from build123d import *

# Parameters (mm, degrees)
BOSS_EXTRUDE1_DEPTH = 7
SKETCH4_R           = 11
CUT_EXTRUDE1_DEPTH  = 8
SKETCH7_R           = 4
CUT_EXTRUDE2_DEPTH  = 8


with BuildPart() as part:
    # Sketch2 → Boss-Extrude1 (new body)
    with BuildSketch(Plane.XY):
        with BuildLine():
            Line((0, 0), (45, 0))
            ThreePointArc((45, 0), (65, 20), (45, 40))
            Line((45, 40), (0, 40))
            ThreePointArc((0, 40), (-20, 20), (0, 0))
        make_face()
    extrude(amount=BOSS_EXTRUDE1_DEPTH)

    # Sketch4 → Cut-Extrude1 (cut, through all)
    with BuildSketch(Plane(origin=(0, 0, 0), x_dir=(-1, 0, 0), z_dir=(0, 0, -1))):
        with Locations((0, 20)):
            Circle(SKETCH4_R)
    extrude(amount=-CUT_EXTRUDE1_DEPTH, mode=Mode.SUBTRACT)

    # Sketch7 → Cut-Extrude2 (cut, through all)
    with BuildSketch(Plane.XY.offset(7)):
        with Locations((45, 20)):
            Circle(SKETCH7_R)
    extrude(amount=-CUT_EXTRUDE2_DEPTH, mode=Mode.SUBTRACT)


solid = part.part
Could you check a few things on this model? Use its own coordinates, in mm. Coordinates: 2 decimals unless noted, no trailing zeros. Order: outer loops, then holes, each group sorted by start corner. A loop starts at its lowest first (then second) coordinate and runs counter-clockwise, first axis right, second up.
Q1. Please list where these lines run through material, in increasing order: L1, parallel to Y at x = 45, z = 4; L2, parallel to Y at x = 0, z = 2; L3, parallel to X at y = 23.5, z = 5.
Q2. Will this pin go through, and if not, where does the flat tip stop? pin 1 (13 mm diameter, centred on x = 0, y = 20, fed in from -Z).
Q3. Thinking about a two-plate mould opening in Y: for faces 1 (the flat face through (23, 40, 3)), 2 (the flat face through (22, 0, 3)), 3 (the cylindrical face through (42.05, 22.7, 3.55)), which applies, released by +Y, released by -Y, zero draft, split by the parting line, or undercut?
Q4. Suppose I cut it at B-B on z = 1.75. Please give me the cut outline in (x, y), and give its area (3 significant figures).
Q5. Suppose I cut it at D-D on x = -7. Please give me the cut outline in (y, z) (3 decimals).
Q6. Suppose I cut it at C-C on y = 11.5. Please give me the cut outline in (x, z), and give its area (3 significant figures).
Q7. Suppose I cut it at A-A on y = 20. Please give me the cut outline in (x, z), and give its area (3 significant figures).
Answer:
1. L1: y = 0 to 16, 24 to 40
1. L2: y = 0 to 9, 31 to 40
1. L3: x = -19.69 to -10.43, 10.43 to 43.06, 46.94 to 64.69
2. pin 1: passes through
3. face 1: released by +Y
3. face 2: released by -Y
3. face 3: undercut
4. outline: (0, 0) - (45, 0) arc R20 ccw to (45, 40) - (0, 40) arc R20 ccw to start; hole circle Ø22 at (0, 20); hole circle Ø8 at (45, 20)
4. area: 2,630 mm2
5. outline: (1.265, 0) - (11.515, 0) - (11.515, 7) - (1.265, 7) - close; (28.485, 0) - (38.735, 0) - (38.735, 7) - (28.485, 7) - close
6. outline: (-18.1, 0) - (-6.98, 0) - (-6.98, 7) - (-18.1, 7) - close; (6.98, 0) - (63.1, 0) - (63.1, 7) - (6.98, 7) - close
6. area: 471 mm2
7. outline: (-20, 0) - (-11, 0) - (-11, 7) - (-20, 7) - close; (11, 0) - (41, 0) - (41, 7) - (11, 7) - close; (49, 0) - (65, 0) - (65, 7) - (49, 7) - close
7. area: 385 mm2
